Part model, mm, in its own coordinate system. Face numbers are marked on the shaded views. A direction names the side the tool comes from. Coordinates: 2 decimals unless noted, no trailing zeros. Write each loop counter-clockwise with the first axis right and the second up, starting at its lowest first coordinate (ties: lowest second). Pieces come first, ordered by that corner, then holes. Notation, with made-up numbers: (46, 55) - (64, 55) arc R17 ccw to (64, 70) - close; hole circle Ø4 at (67.5, 15.25). An arc over 180 degrees is marked (long way). Write each question's results on one line, items separated by ' | '.
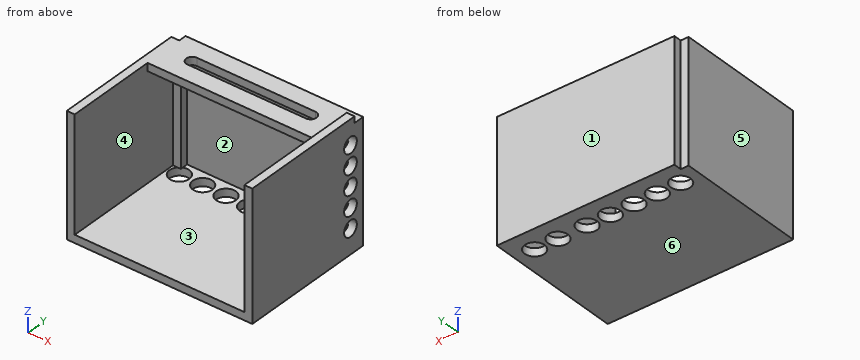
from build123d import *

# Parameters (mm, degrees)
F0_W      = 470
F0_H      = 325
F1_DEPTH  = 350
F2_T      = -20
F3_W      = 27
F3_H      = 16
F4_DEPTH  = 470.001
F5_R      = 25
F6_DEPTH  = 325.001
F7_R      = 20
F8_DEPTH  = 20
F9_W      = 20
F9_H      = 16
F10_DEPTH = 323.001
F11_W     = 20
F11_H     = 20
F12_DEPTH = 289
F13_W     = 20
F13_H     = 20
F14_DEPTH = 309.001
F15_W     = 100
F15_H     = 20
F16_DEPTH = 430
F18_DEPTH = 20


with BuildPart() as f1:
    # F0 (on Front) → F1 (new body)
    with BuildSketch(Plane.XZ):
        with Locations((235, 162.5)):
            Rectangle(F0_W, F0_H)
    extrude(amount=F1_DEPTH)

    # F2
    f2_openings = [f1.faces().sort_by_distance(p)[0] for p in [
        (235, -350, 162.5),
        (235, -175, 325),
    ]]
    offset(amount=F2_T, openings=f2_openings)

    # F3 (on face) → F4 (cut, through all)
    with BuildSketch(Plane.YZ.offset(470)):
        with Locations((-13.5, 317)):
            Rectangle(F3_W, F3_H)
    extrude(amount=-F4_DEPTH, mode=Mode.SUBTRACT)

    # F5 (on Top) → F6 (cut, through all)
    with BuildSketch(Plane.XY):
        with Locations((50, -57)):
            Circle(F5_R)
        with Locations((109, -57)):
            Circle(F5_R)
        with Locations((168, -57)):
            Circle(F5_R)
        with Locations((361, -57)):
            Circle(F5_R)
        with Locations((420, -57)):
            Circle(F5_R)
        with Locations((228, -57)):
            Circle(F5_R)
        with Locations((287, -57)):
            Circle(F5_R)
    extrude(amount=F6_DEPTH, mode=Mode.SUBTRACT)

    # F7 (on face) → F8 (cut, through all)
    with BuildSketch(Plane.YZ.offset(470)):
        with Locations((-40, 62.5)):
            Circle(F7_R)
        with BuildLine():
            ThreePointArc((-60, 162.5), (-40, 142.5), (-20, 162.5))
            ThreePointArc((-20, 162.5), (-40, 182.5), (-60, 162.5))
        make_face()
        with Locations((-40, 212.5)):
            Circle(F7_R)
        with Locations((-40, 262.5)):
            Circle(F7_R)
        with Locations((-40, 112.5)):
            Circle(F7_R)
    extrude(amount=-F8_DEPTH, mode=Mode.SUBTRACT)

    # F9 (on face) → F10 (cut, through all)
    with BuildSketch(Plane(origin=(0, -27, 0), x_dir=(-1, 0, 0), z_dir=(0, 1, 0))):
        with Locations((-10, 317)):
            Rectangle(F9_W, F9_H)
    extrude(amount=-F10_DEPTH, mode=Mode.SUBTRACT)

    # F11 (on face) → F12 (join, through all)
    with BuildSketch(Plane.XY.offset(309)):
        with Locations((30, -30)):
            Rectangle(F11_W, F11_H)
    extrude(amount=-F12_DEPTH)

    # F13 (on face) → F14 (cut, through all)
    with BuildSketch(Plane.XY.offset(309)):
        with Locations((10, -10)):
            Rectangle(F13_W, F13_H)
    extrude(amount=-F14_DEPTH, mode=Mode.SUBTRACT)

    # F15 (on face) → F16 (join, through all)
    with BuildSketch(Plane.YZ.offset(20)):
        with Locations((-70, 299)):
            Rectangle(F15_W, F15_H)
    extrude(amount=F16_DEPTH)

    # F17 (on face) → F18 (cut, through all)
    with BuildSketch(Plane.XY.offset(309)):
        with BuildLine():
            Line((85, -60), (85, -45))
            ThreePointArc((85, -45), (70, -60), (85, -75))
            Line((85, -75), (85, -60))
        make_face()
        Polygon((235, -45), (85, -45), (85, -60), (85, -75), (235, -75), align=None)
        with BuildLine():
            Line((385, -45), (235, -45))
            Line((235, -45), (235, -75))
            Line((235, -75), (385, -75))
            ThreePointArc((385, -75), (400, -60), (385, -45))
        make_face()
    extrude(amount=-F18_DEPTH, mode=Mode.SUBTRACT)


solid = f1.part
(1) Saw through at B-B on x = 50. Write the cut outline in (y, z).
Return value:
outline: (-350, 0) - (-82, 0) - (-82, 20) - (-350, 20) - close; (-120, 289) - (-20, 289) - (-20, 20) - (-32, 20) - (-32, 0) - (0, 0) - (0, 309) - (-120, 309) - close
(2) Two-plate mould, pull along Z, no slides. Class the marked faces 3, 4, 5 and 6: released by +Z, released by -Z, zero draft, split by the parting line, or undercut.
Return value:
face 3: undercut | face 4: undercut | face 5: zero draft | face 6: released by -Z
(3) Flat gauge pins, fed straight in: P1, Ø1.5, axis at x = 342.5, z = 84, coming from the -Y side; P2, Ø6, axis at x = 285, z = 294, coming from the +Y side; P3, Ø22, axis at x = 279, z = 295.5, coming from the -Y side; P4, Ø13, axis at x = 458, z = 318.5, coming from the +Y side. Where does each tip first touch, or does it go through?
Return value:
P1: stops at y = -20 | P2: stops at y = 0 | P3: stops at y = -120 | P4: stops at y = -27
(4) Wall check: line 1 (Z direction, x = 464, y = -40); line 2 (Y direction, x = 287, z = 12); line 3 (X direction, y = -89.5, z = 107). Give the ranges that are in metal, low to high. Write a range as from..to.
Return value:
line 1: z = 0..42.5, 82.5..92.5, 132.5..142.5, 182.5..192.5, 232.5..242.5, 282.5..325 | line 2: y = -350..-82, -32..0 | line 3: x = 0..20, 450..470
(5) 3-axis set-ups, long thin cutter, end or side, ignore diameter. For the marked faces 1 and 2: which of +Z, -Z, +X, -X, +Y, -Y reach the whole face in a straight line?
Return value:
face 1: +Z, -Z, +X, -X, +Y | face 2: -Y
(6) Saw through at A-A on z = 295. Write the cut outline in (x, y), then the cut area to 3 significant figures.
Return value:
outline: (0, -350) - (20, -350) - (20, -120) - (450, -120) - (450, -350) - (470, -350) - (470, 0) - (20, 0) - (20, -20) - (0, -20) - close; hole (85, -75) - (385, -75) arc R15 ccw to (385, -45) - (85, -45) arc R15 ccw to start | area: 55,500 mm^2
(7) Saw through at D-D on x = 109. Write the cut outline in (y, z).
Return value:
outline: (-350, 0) - (-82, 0) - (-82, 20) - (-350, 20) - close; (-120, 289) - (-75, 289) - (-75, 309) - (-120, 309) - close; (-45, 289) - (-20, 289) - (-20, 20) - (-32, 20) - (-32, 0) - (0, 0) - (0, 309) - (-45, 309) - close
(8) Saw through at C-C on y = -325. Write the cut outline in (x, z).
Return value:
outline: (0, 0) - (470, 0) - (470, 325) - (450, 325) - (450, 20) - (20, 20) - (20, 309) - (0, 309) - close
